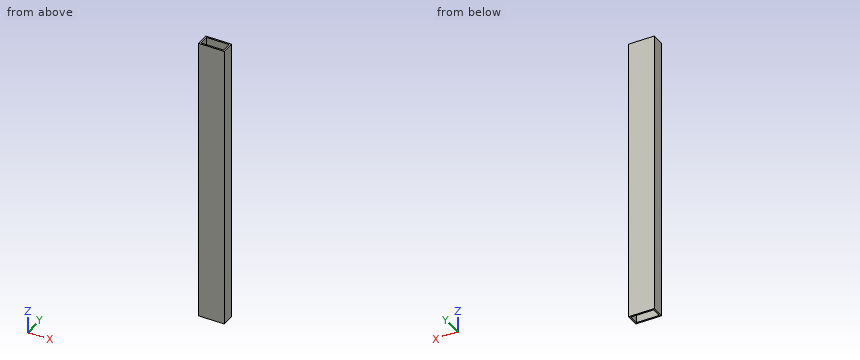
```python
from build123d import *

# Parameters (mm, degrees)
BOSS_EXTRUDE1_START = 3.175
SKETCH1_W           = 50.8
SKETCH1_H           = 25.4
SKETCH1_W_2         = 44.704
SKETCH1_H_2         = 19.304
BOSS_EXTRUDE1_DEPTH = 555.625


with BuildPart() as part:
    # Sketch1 → Boss-Extrude1 (new body)
    with BuildSketch(Plane.XY.offset(BOSS_EXTRUDE1_START)):
        with Locations((25.4, 12.7)):
            Rectangle(SKETCH1_W, SKETCH1_H)
        with Locations((25.4, 12.7)):
            Rectangle(SKETCH1_W_2, SKETCH1_H_2, mode=Mode.SUBTRACT)
    extrude(amount=BOSS_EXTRUDE1_DEPTH)


solid = part.part
```
Geometry: final body of the model. Coordinates: model frame, mm. Give positions to 0.01 mm unless a question says otherwise; leave off trailing zeros. Loops run counter-clockwise (first coordinate to the right, second up) from the corner with the lowest first, then second, coordinate; pieces in that order, holes last. Notation, with made-up numbers: (15.25, -32) -> (50.25, -32) arc R8 ccw to (50.25, -27) -> close; hole circle Ø11 at (85.5, 34). An arc over 180 degrees is marked (long way). Use one line per item in the form item = value.
Item 1: Section query C-C on z = 48. Output: boundary loops of the cut face in (x, y), and give its area (3 significant figures).
A:
outline = (0, 0) -> (50.8, 0) -> (50.8, 25.4) -> (0, 25.4) -> close; hole (3.05, 3.05) -> (47.75, 3.05) -> (47.75, 22.35) -> (3.05, 22.35) -> close
area = 427 mm^2
Item 2: Section query B-B on x = 9.5. Output: boundary loops of the cut face in (y, z) (3 decimals), and give its area (3 significant figures).
A:
outline = (0, 3.175) -> (3.048, 3.175) -> (3.048, 558.8) -> (0, 558.8) -> close; (22.352, 3.175) -> (25.4, 3.175) -> (25.4, 558.8) -> (22.352, 558.8) -> close
area = 3,390 mm^2
Item 3: Line query: probe 1 along Y at (x, z) = (12.5, 350.5); probe 2 along X at (y, z) = (14.75, 416). Output: solid intervals per line, ascending.
A:
probe_1 = 0 to 3.05, 22.35 to 25.4
probe_2 = 0 to 3.05, 47.75 to 50.8
Item 4: Section query A-A on y = 7.25. Output: boundary loops of the cut face in (x, z) (3 decimals).
A:
outline = (0, 3.175) -> (3.048, 3.175) -> (3.048, 558.8) -> (0, 558.8) -> close; (47.752, 3.175) -> (50.8, 3.175) -> (50.8, 558.8) -> (47.752, 558.8) -> close
